Part model, mm, in its own coordinate system. Round coordinates to 2 decimals unless told otherwise and drop trailing zeros. Write each loop counter-clockwise with the first axis right and the second up, starting at its lowest first coordinate (ties: lowest second). Pieces come first, ordered by that corner, then holes.
```python
from build123d import *

# Parameters (mm, degrees)
SKETCH1_W           = 30
SKETCH1_H           = 3
SKETCH1_W_2         = 3
SKETCH1_H_2         = 30
BOSS_EXTRUDE1_DEPTH = 3
CUT_EXTRUDE1_DEPTH  = 10


with BuildPart() as part:
    # Sketch1 → Boss-Extrude1 (new body)
    with BuildSketch(Plane(origin=(0, 0, 0), x_dir=(1, 0, 0), z_dir=(0, 1, 0))):
        with Locations((0, -56)):
            Rectangle(SKETCH1_W, SKETCH1_H)
        with Locations((-56, 0)):
            Rectangle(SKETCH1_W_2, SKETCH1_H_2)
        with Locations((0, 56)):
            Rectangle(SKETCH1_W, SKETCH1_H)
        Polygon((-54.5, -54.5), (-54.5, -15), (-54.5, 15), (-54.5, 54.5), (-15, 54.5), (15, 54.5), (54.5, 54.5), (54.5, 15), (54.5, -15), (54.5, -54.5), (15, -54.5), (-15, -54.5), align=None)
        with Locations((56, 0)):
            Rectangle(SKETCH1_W_2, SKETCH1_H_2)
    extrude(amount=BOSS_EXTRUDE1_DEPTH)

    # Sketch2 → Cut-Extrude1 (cut)
    with BuildSketch(Plane(origin=(0, 3, 0), x_dir=(1, 0, 0), z_dir=(0, 1, 0))):
        Polygon((-15, -30.5), (-15, -27.5), (15, -27.5), (15, -30.499716912), (54.5, -30.499716912), (54.5, -57.5), (-54.5, -57.5), (-54.5, -30.5), align=None)
    extrude(amount=-CUT_EXTRUDE1_DEPTH, mode=Mode.SUBTRACT)


solid = part.part
```
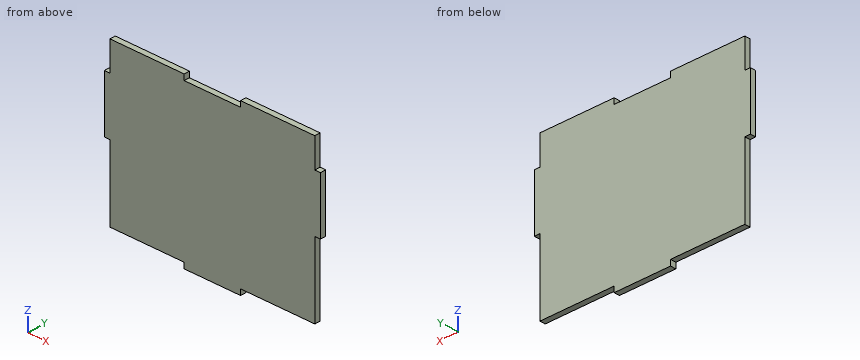
Q1. Cut at B-B on x = -31.5. Write the cut outline in (y, z).
Values follow:
outline: (0, -54.5) - (3, -54.5) - (3, 30.5) - (0, 30.5) - close
Q2. Cut at A-A on y = 1.8. Write the cut outline in (x, z).
Values follow:
outline: (-57.5, -15) - (-54.5, -15) - (-54.5, -54.5) - (-15, -54.5) - (-15, -57.5) - (15, -57.5) - (15, -54.5) - (54.5, -54.5) - (54.5, -15) - (57.5, -15) - (57.5, 15) - (54.5, 15) - (54.5, 30.5) - (15, 30.5) - (15, 27.5) - (-15, 27.5) - (-15, 30.5) - (-54.5, 30.5) - (-54.5, 15) - (-57.5, 15) - close
Q3. Drop flat-ended pins along their axis: pin 1 (0.9 mm diameter, centred on x = -55.5, y = 1.5, fed in from -Z); pin 2 (1.5 mm diameter, centred on y = 1, z = 28.5, fed in from -X); pin 3 (0.9 mm diameter, centred on y = 2, z = -36, fed in from +X). Give the stop position or say it passes through.
Values follow:
pin 1: stops at z = -15
pin 2: stops at x = -54.5
pin 3: stops at x = 54.5
Q4. Wall check: L1, parallel to Z at x = 17, y = 0.4; L2, parallel to X at y = 0.4, z = -47; L3, parallel to Z at x = -6.5, y = 1.95. Give the ranges that are in metal, low to high.
Values follow:
L1: z = -54.5 to 30.5
L2: x = -54.5 to 54.5
L3: z = -57.5 to 27.5
Q5. Cut at C-C on z = -35. Write the cut outline in (x, y), plus the area to 3 significant figures.
Values follow:
outline: (-54.5, 0) - (54.5, 0) - (54.5, 3) - (-54.5, 3) - close
area: 327 mm2
